Work out the finished part from the listing and answer in its coordinate system (mm). Face numbers are marked on the shaded views. A direction names the side the tool comes from. Coordinates: 2 decimals unless noted, no trailing zeros. Loops run counter-clockwise (first coordinate to the right, second up) from the corner with the lowest first, then second, coordinate; pieces in that order, holes last. Notation, with made-up numbers: (51.5, 29) -> (89.5, 29) arc R13 cw to (89.5, 41) -> close; hole circle Ø5 at (89, 44.25). An arc over 180 degrees is marked (long way). Use a Markdown table: item, result.
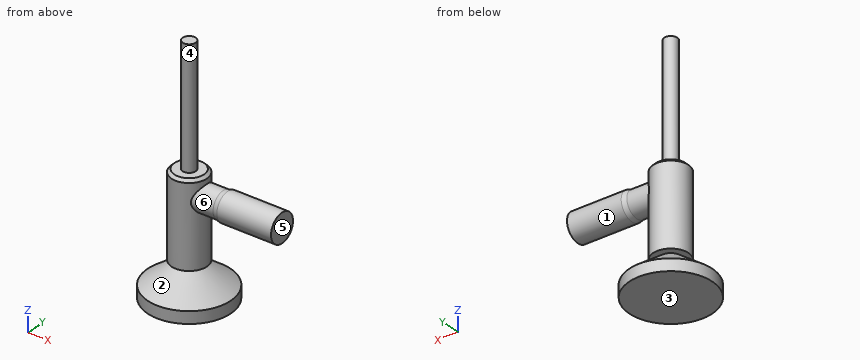
from build123d import *

# Parameters (mm, degrees)
ESQUISSE1_R        = 17.5
BOSS_EXTRU_1_DEPTH = 5
ESQUISSE2_R        = 17.5
BOSS_EXTRU_2_DEPTH = 9.7
CHANFREIN1_SIZE    = 9.7
CHANFREIN1_SIZE2   = 13.05
ESQUISSE3_R        = 7.45
BOSS_EXTRU_3_DEPTH = 35.4
ESQUISSE4_R        = 2.75
BOSS_EXTRU_4_DEPTH = 50
ESQUISSE5_R        = 5.5
BOSS_EXTRU_5_DEPTH = 14.4
CHANFREIN2_SIZE    = 1.19
ESQUISSE6_R        = 6
BOSS_EXTRU_6_DEPTH = 25
CHANFREIN3_SIZE2   = 0.5
CHANFREIN3_SIZE    = 2


with BuildPart() as part:
    # Esquisse1 → Boss.-Extru.1 (new body)
    with BuildSketch(Plane.XY):
        Circle(ESQUISSE1_R)
    extrude(amount=BOSS_EXTRU_1_DEPTH)

    # Esquisse2 → Boss.-Extru.2 (add)
    with BuildSketch(Plane.XY.offset(5)):
        Circle(ESQUISSE2_R)
    extrude(amount=BOSS_EXTRU_2_DEPTH)

    # Chanfrein1
    chanfrein1_edges = [part.edges().sort_by_distance(p)[0] for p in [
        (-17.5, 0, 14.7),
    ]]
    chanfrein1_side = [part.faces().sort_by_distance(p)[0] for p in [
        (-17.5, 0, 7.35),
    ]]
    chamfer(chanfrein1_edges, length=CHANFREIN1_SIZE, length2=CHANFREIN1_SIZE2, reference=chanfrein1_side[0])

    # Esquisse3 → Boss.-Extru.3 (add)
    with BuildSketch(Plane.XY.offset(14.7)):
        Circle(ESQUISSE3_R)
    extrude(amount=BOSS_EXTRU_3_DEPTH)

    # Esquisse4 → Boss.-Extru.4 (add)
    with BuildSketch(Plane.XY.offset(50.1)):
        Circle(ESQUISSE4_R)
    extrude(amount=BOSS_EXTRU_4_DEPTH)

    # Esquisse5 → Boss.-Extru.5 (add)
    with BuildSketch(Plane(origin=(0, 0, 0), x_dir=(0, 0, -1), z_dir=(1, 0, 0))):
        with Locations((-41.3, 0)):
            Circle(ESQUISSE5_R)
    extrude(amount=BOSS_EXTRU_5_DEPTH)

    # Chanfrein2
    chanfrein2_edges = [part.edges().sort_by_distance(p)[0] for p in [
        (-7.45, 0, 50.1),
    ]]
    chamfer(chanfrein2_edges, length=CHANFREIN2_SIZE)

    # Esquisse6 → Boss.-Extru.6 (add)
    with BuildSketch(Plane(origin=(14.4, 0, 0), x_dir=(0, 0, -1), z_dir=(1, 0, 0))):
        with Locations((-41.3, 0)):
            Circle(ESQUISSE6_R)
    extrude(amount=BOSS_EXTRU_6_DEPTH)

    # Chanfrein3
    chanfrein3_edges = [part.edges().sort_by_distance(p)[0] for p in [
        (14.4, 0, 47.3),
    ]]
    chanfrein3_side = [part.faces().sort_by_distance(p)[0] for p in [
        (14.41, 0, 47.3),
    ]]
    chamfer(chanfrein3_edges, length=CHANFREIN3_SIZE - 0.0001, length2=CHANFREIN3_SIZE2 - 0.0001, reference=chanfrein3_side[0])  # a hair under: the kernel refuses the full size


solid = part.part
Q1. For the marked faces 1 and 2, determine the directions among +Z, -Z, +X, -X, +Y, -Y from which every point of the face is accessible in a straight line to the end or side of a thin tool.
Solved:
| item | result |
|---|---|
| face 1 | +X |
| face 2 | none |
Q2. Section D-D on z = 66.5 is taken. Determine the outline of the cut face in (x, y).
Solved:
| item | result |
|---|---|
| outline | circle Ø5.5 at (0, 0) |
Q3. Consider line 1 (Z direction, x = -9, y = -6); line 2 (Z direction, x = 11, y = -10); line 3 (X direction, y = 1, z = 48.5). Determine where each line is inside the solid, lowest interval first. Write a range as [from, to].
Solved:
| item | result |
|---|---|
| line 1 | [0, 9.97] |
| line 2 | [0, 6.96] |
| line 3 | [-7.38, 7.38] |
Q4. Given pin 1 Ø4 at (x, y) = (13.5, 6) entering from +Z; pin 2 Ø10 at (x, z) = (-3.5, 30.5) entering from -Y; pin 3 Ø8 at (y, z) = (-5, 55.5) entering from +X; pin 4 Ø6 at (x, z) = (23, 51) entering from -Y, each flat-ended and moving along its own axis, determine where each tip first touches the part or whether it passes through.
Solved:
| item | result |
|---|---|
| pin 1 | z = 45.07 |
| pin 2 | y = -7.45 |
| pin 3 | x = 2.56 |
| pin 4 | through |
Q5. Section B-B on x = 0 is taken. Determine the outline of the cut face in (y, z), and give its area (3 significant figures).
Solved:
| item | result |
|---|---|
| outline | (-17.5, 0) -> (17.5, 0) -> (17.5, 5) -> (4.45, 14.7) -> (7.45, 14.7) -> (7.45, 48.91) -> (6.26, 50.1) -> (2.75, 50.1) -> (2.75, 100.1) -> (-2.75, 100.1) -> (-2.75, 50.1) -> (-6.26, 50.1) -> (-7.45, 48.91) -> (-7.45, 14.7) -> (-4.45, 14.7) -> (-17.5, 5) -> close |
| area | 1,190 mm² |
Q6. Determine the mould class of the marked faces 3, 4, 5 and 6 for opening direction X: pulls with the +X half, pulls with the -X half, needs draft (parallel to the pull), parting line crosses it, or undercut.
Solved:
| item | result |
|---|---|
| face 3 | needs draft |
| face 4 | parting line crosses it |
| face 5 | pulls with the +X half |
| face 6 | undercut |
